Can you work these out from the model? Positions are in its coordinate system, mm. A direction names the side the tool comes from. Give positions to 0.01 mm unless a question says otherwise; leave off trailing zeros. Loops run counter-clockwise (first coordinate to the right, second up) from the corner with the lowest first, then second, coordinate; pieces in that order, holes last. Notation, with made-up numbers: M 1,12 L 31,12 A28 cw 31,49 Z; hole C 54.25,5 d7. An arc over 180 degrees is marked long. Use CSV: the item, a comma, the result in double quotes.
from build123d import *

# Parameters (mm, degrees)
SKETCH315_W     = 60
SKETCH315_H     = 45
PAD148_DEPTH    = 5
SKETCH318_W     = 64
SKETCH318_H     = 49
SKETCH318_W_2   = 60
SKETCH318_H_2   = 45
PAD149_DEPTH    = 20
SKETCH319_W     = 62
SKETCH319_H     = 47
PAD150_DEPTH    = 1
PAD151_DEPTH    = 2
SKETCH316_W     = 18
SKETCH316_H     = 4
POCKET130_DEPTH = 5.5
SKETCH317_R     = 2.25
POCKET131_DEPTH = 5
SKETCH323_R     = 3.75
POCKET132_DEPTH = 3.5
SKETCH324_W     = 3
SKETCH324_H     = 16
POCKET133_DEPTH = 5
SKETCH325_W     = 5
SKETCH325_H     = 18
SKETCH325_W_2   = 3
SKETCH325_H_2   = 16
PAD152_DEPTH    = 2
SKETCH321_R     = 3
PAD153_DEPTH    = 3
SKETCH322_R     = 1.5
POCKET134_DEPTH = 5
SKETCH326_R     = 3
PAD154_DEPTH    = 3
SKETCH327_R     = 1
POCKET135_DEPTH = 5
POCKET136_DEPTH = 5
PAD155_DEPTH    = 2
SKETCH330_R     = 2.5
POCKET137_DEPTH = 5
SKETCH331_R     = 5.5
SKETCH331_R_2   = 2.5
PAD156_DEPTH    = 2


with BuildPart() as part:
    # Sketch315 → Pad148 (new body)
    with BuildSketch(Plane.XY):
        with BuildLine():
            Line((-32, 24.5), (-20, 24.5))
            Line((-20, 24.5), (-20, 37.5))
            ThreePointArc((-10, 37.5), (-15, 42.5), (-20, 37.5))
            Line((-10, 24.5), (-10, 37.5))
            Line((-10, 24.5), (27.428932, 24.5))
            Line((27.428932, 24.5), (31.464466, 28.535534))
            ThreePointArc((38.535534, 21.464466), (38.535534, 28.535534), (31.464466, 28.535534))
            Line((32, 14.928932), (38.535534, 21.464466))
            Line((32, 14.928932), (32, -14.928932))
            Line((32, -14.928932), (38.535534, -21.464466))
            ThreePointArc((31.464466, -28.535534), (38.535534, -28.535534), (38.535534, -21.464466))
            Line((27.428932, -24.5), (31.464466, -28.535534))
            Line((27.428932, -24.5), (-10, -24.5))
            Line((-10, -24.5), (-10, -37.5))
            ThreePointArc((-20, -37.5), (-15, -42.5), (-10, -37.5))
            Line((-20, -24.5), (-20, -37.5))
            Line((-20, -24.5), (-32, -24.5))
            Line((-32, -24.5), (-32, 24.5))
        make_face()
        Rectangle(SKETCH315_W, SKETCH315_H, mode=Mode.SUBTRACT)
    extrude(amount=PAD148_DEPTH)

    # Sketch318 → Pad149 (join)
    with BuildSketch(Plane.XY):
        Rectangle(SKETCH318_W, SKETCH318_H)
        Rectangle(SKETCH318_W_2, SKETCH318_H_2, mode=Mode.SUBTRACT)
    extrude(amount=-PAD149_DEPTH)

    # Sketch319 (on Face13 of Pad149) → Pad150 (join)
    with BuildSketch(Plane(origin=(0, 0, -20), x_dir=(1, 0, 0), z_dir=(0, 0, -1))):
        Rectangle(SKETCH319_W, SKETCH319_H)
    extrude(amount=-PAD150_DEPTH)

    # Sketch320 (on Face38 of Pad150) → Pad151 (join)
    with BuildSketch(Plane(origin=(0, 0, -20), x_dir=(1, 0, 0), z_dir=(0, 0, -1))):
        Polygon((-31, 1), (-17, 1), (-17, 23.5), (-15, 23.5), (-15, 1), (-1, 1), (-1, 23.5), (1, 23.5), (1, 1), (15, 1), (15, 23.5), (17, 23.5), (17, 1), (31, 1), (31, -1), (17, -1), (17, -23.5), (15, -23.5), (15, -1), (1, -1), (1, -23.5), (-1, -23.5), (-1, -1), (-15, -1), (-15, -23.5), (-17, -23.5), (-17, -1), (-31, -1), align=None)
    extrude(amount=-PAD151_DEPTH)

    # Sketch316 → Pocket130 (cut, symmetric)
    with BuildSketch(Plane(origin=(30, 0, 0), x_dir=(0, -1, 0), z_dir=(-1, 0, 0))):
        with Locations((-10, 1)):
            Rectangle(SKETCH316_W, SKETCH316_H)
        with Locations((10, 1)):
            Rectangle(SKETCH316_W, SKETCH316_H)
    extrude(amount=POCKET130_DEPTH, both=True, mode=Mode.SUBTRACT)

    # Sketch317 → Pocket131 (cut)
    with BuildSketch(Plane.XY):
        with Locations((35, -25)):
            Circle(SKETCH317_R)
        with Locations((35, 25)):
            Circle(SKETCH317_R)
        with Locations((-15, 37.5)):
            Circle(SKETCH317_R)
        with Locations((-15, -37.5)):
            Circle(SKETCH317_R)
        with BuildLine():
            Line((-17, 24.5), (-13, 24.5))
            Line((-13, 24.5), (-13, 32.917424))
            ThreePointArc((-17, 32.917424), (-15, 32.5), (-13, 32.917424))
            Line((-17, 24.5), (-17, 32.917424))
        make_face()
        with BuildLine():
            Line((-17, -24.5), (-13, -24.5))
            Line((-13, -24.5), (-13, -32.917424))
            ThreePointArc((-13, -32.917424), (-15, -32.5), (-17, -32.917424))
            Line((-17, -24.5), (-17, -32.917424))
        make_face()
    extrude(amount=POCKET131_DEPTH, mode=Mode.SUBTRACT)

    # Sketch323 → Pocket132 (cut)
    with BuildSketch(Plane.XY):
        with Locations((35, -25)):
            Circle(SKETCH323_R)
        with Locations((35, 25)):
            Circle(SKETCH323_R)
        with Locations((-15, 37.5)):
            Circle(SKETCH323_R)
        with Locations((-15, -37.5)):
            Circle(SKETCH323_R)
    extrude(amount=POCKET132_DEPTH, mode=Mode.SUBTRACT)

    # Sketch324 (on Face87 of Pocket132) → Pocket133 (cut)
    with BuildSketch(Plane(origin=(0, 0, -20), x_dir=(1, 0, 0), z_dir=(0, 0, -1))):
        with Locations((-27.5, 0)):
            Rectangle(SKETCH324_W, SKETCH324_H)
    extrude(amount=-POCKET133_DEPTH, mode=Mode.SUBTRACT)

    # Sketch325 (on Face87 of Pocket133) → Pad152 (join)
    with BuildSketch(Plane(origin=(0, 0, -20), x_dir=(1, 0, 0), z_dir=(0, 0, -1))):
        with Locations((-27.5, 0)):
            Rectangle(SKETCH325_W, SKETCH325_H)
        with Locations((-27.5, 0)):
            Rectangle(SKETCH325_W_2, SKETCH325_H_2, mode=Mode.SUBTRACT)
    extrude(amount=-PAD152_DEPTH)

    # Sketch321 (on Face13 of Pad151) → Pad153 (join)
    with BuildSketch(Plane(origin=(0, 0, -20), x_dir=(1, 0, 0), z_dir=(0, 0, -1))):
        with Locations((-16, 16)):
            Circle(SKETCH321_R)
        with Locations((-16, -16)):
            Circle(SKETCH321_R)
    extrude(amount=-PAD153_DEPTH)

    # Sketch322 → Pocket134 (cut)
    with BuildSketch(Plane(origin=(0, 0, -20), x_dir=(1, 0, 0), z_dir=(0, 0, -1))):
        with Locations((-16, 16)):
            Circle(SKETCH322_R)
        with Locations((-16, -16)):
            Circle(SKETCH322_R)
    extrude(amount=-POCKET134_DEPTH, mode=Mode.SUBTRACT)

    # Sketch326 (on Face87 of Pad152) → Pad154 (join)
    with BuildSketch(Plane(origin=(0, 0, -20), x_dir=(1, 0, 0), z_dir=(0, 0, -1))):
        with Locations((0, 8)):
            Circle(SKETCH326_R)
        with Locations((0, -8)):
            Circle(SKETCH326_R)
    extrude(amount=-PAD154_DEPTH)

    # Sketch327 → Pocket135 (cut)
    with BuildSketch(Plane(origin=(0, 0, -20), x_dir=(1, 0, 0), z_dir=(0, 0, -1))):
        with Locations((0, 8)):
            Circle(SKETCH327_R)
        with Locations((0, -8)):
            Circle(SKETCH327_R)
    extrude(amount=-POCKET135_DEPTH, mode=Mode.SUBTRACT)

    # Sketch328 (on Face15 of Pocket135) → Pocket136 (cut)
    with BuildSketch(Plane(origin=(0, 0, -20), x_dir=(1, 0, 0), z_dir=(0, 0, -1))):
        with BuildLine():
            ThreePointArc((26, 19), (24, 21), (22, 19))
            Line((22, -19), (22, 19))
            ThreePointArc((22, -19), (24, -21), (26, -19))
            Line((26, -19), (26, 19))
        make_face()
    extrude(amount=-POCKET136_DEPTH, mode=Mode.SUBTRACT)

    # Sketch329 (on Face15 of Pocket135) → Pad155 (join)
    with BuildSketch(Plane(origin=(0, 0, -20), x_dir=(1, 0, 0), z_dir=(0, 0, -1))):
        with BuildLine():
            ThreePointArc((28, 19), (24, 23), (20, 19))
            Line((20, 19), (20, -19))
            ThreePointArc((20, -19), (24, -23), (28, -19))
            Line((28, -19), (28, 19))
        make_face()
        with BuildLine():
            ThreePointArc((26, 19), (24, 21), (22, 19))
            Line((22, -19), (22, 19))
            ThreePointArc((22, -19), (24, -21), (26, -19))
            Line((26, -19), (26, 19))
        make_face(mode=Mode.SUBTRACT)
    extrude(amount=-PAD155_DEPTH)

    # Sketch330 (on Face15 of Pad155) → Pocket137 (cut)
    with BuildSketch(Plane(origin=(0, 0, -20), x_dir=(1, 0, 0), z_dir=(0, 0, -1))):
        with Locations((11, 16.5)):
            Circle(SKETCH330_R)
    extrude(amount=-POCKET137_DEPTH, mode=Mode.SUBTRACT)

    # Sketch331 (on Face15 of Pocket137) → Pad156 (join)
    with BuildSketch(Plane(origin=(0, 0, -20), x_dir=(1, 0, 0), z_dir=(0, 0, -1))):
        with Locations((11, 16.5)):
            Circle(SKETCH331_R)
        with Locations((11, 16.5)):
            Circle(SKETCH331_R_2, mode=Mode.SUBTRACT)
    extrude(amount=-PAD156_DEPTH)


with BuildPart() as part_1:
    # Body033 placement: moved
    add(part.part.moved(Location((-216, 0, 0))))


solid = part_1.part
Q1. I'm going to push flat-ended pins straight in: P1, Ø1.5, axis at x = -204.5, z = -11, coming from the -Y side; P2, Ø5, axis at x = -231, y = -37.5, coming from the -Z side; P3, Ø2.5, axis at y = -29.5, z = 2, coming from the -X side. Where does each tip first touch, or does it pass through?
Model answer:
P1,"y = -24.5"
P2,"z = 3.5"
P3,"x = -236"
Q2. If we mould it in two halves opening along Y, with no side actions, what happens to faces 4 (the flat face through (-231, -33, 0)), 5 (the flat face through (-233, -29, 2))? For each: released by +Y, released by -Y, zero draft, split by the parting line, or undercut.
Model answer:
face 4,"zero draft"
face 5,"undercut"
Q3. I want a section at C-C, the plane x = -204. Please give me the cut outline in (y, z), then the cut area to 3 significant figures.
Model answer:
outline,"M -24.5,-20 L -18.79,-20 L -18.79,-18 L -21.91,-18 L -21.91,-19 L -22.5,-19 L -22.5,5 L -24.5,5 Z; M -14.21,-20 L 24.5,-20 L 24.5,5 L 22.5,5 L 22.5,-19 L 1,-19 L 1,-18 L -1,-18 L -1,-19 L -11.09,-19 L -11.09,-18 L -14.21,-18 Z"
area,"149 mm2"
Q4. I want a section at B-B, the plane z = -11.25. Please give me the cut outline in (x, y).
Model answer:
outline,"M -248,-24.5 L -184,-24.5 L -184,24.5 L -248,24.5 Z; hole M -246,-22.5 L -186,-22.5 L -186,22.5 L -246,22.5 Z"
Q5. For faces 1 (the flat face through (-226, -31, 2)), 2 (the flat face through (-208, 12, -19)), 3 (the flat face through (-180.05, 18.88, 3.02)), which set-ups out of +Z, -Z, +X, -X, +Y, -Y let a thin tool reach every point of the face, with its end or its side?
Model answer:
face 1,"+Z, -Z, -Y"
face 2,"+Z"
face 3,"+Z, -Z, +X"
Q6. I want a section at A-A, the plane x = -192. Please give me the cut outline in (y, z), then the cut area to 3 significant figures.
Model answer:
outline,"M -24.5,-20 L -21,-20 L -21,-18 L -22.5,-18 L -22.5,5 L -24.5,5 Z; M 21,-20 L 24.5,-20 L 24.5,5 L 22.5,5 L 22.5,-18 L 21,-18 Z"
area,"106 mm2"
Q7. Please list where these lines run through material, in increasing order: L1, parallel to Y at x = -231, z = 0.85; L2, parallel to Y at x = -232, z = -17.8; L3, parallel to X at y = -7.5, z = -16.5. Write a range as from..to.
Model answer:
L1,"-42.5..-41.25, -33.75..-32.5, -24.5..-22.5, 22.5..24.5, 32.5..33.75, 41.25..42.5"
L2,"-24.5..-22.5, -19..-17.5, -14.5..-13, 13..14.5, 17.5..19, 22.5..24.5"
L3,"-248..-246, -186..-184"
